```python
from build123d import *

# Parameters (mm, degrees)
F0_W     = 431.8
F0_H     = 228.6
F1_DEPTH = 12.7
F3_DEPTH = 22.225
F4_W     = 3.175
F4_H     = 12.7
F5_DEPTH = 203.2


with BuildPart() as f1:
    # F0 (on Front) → F1 (new body)
    with BuildSketch(Plane.XZ):
        with Locations((215.9, 114.3)):
            Rectangle(F0_W, F0_H)
    extrude(amount=F1_DEPTH)

    # F2 (on face) → F3 (join)
    with BuildSketch(Plane.XZ.offset(12.7)):
        Polygon((139.7, 107.95), (139.7, 114.3), (139.7, 120.65), (114.3, 120.65), (114.3, 114.3), (114.3, 107.95), align=None)
        Polygon((317.5, 120.65), (292.1, 120.65), (292.1, 114.3), (292.1, 107.95), (317.5, 107.95), (317.5, 114.3), align=None)
    extrude(amount=F3_DEPTH)

    # F4 (on face) → F5 (join, through all)
    with BuildSketch(Plane.YZ.offset(317.5)):
        with Locations((-36.5125, 114.3)):
            Rectangle(F4_W, F4_H)
    extrude(amount=-F5_DEPTH)


solid = f1.part
```
The listing builds one solid part. Answer for the finished solid, in the listing's coordinates (mm). A direction names the side the tool comes from. Give positions to 0.01 mm unless a question says otherwise; leave off trailing zeros. Order: outer loops, then holes, each group sorted by start corner. A loop starts at its lowest first (then second) coordinate and runs counter-clockwise, first axis right, second up.
Item 1: For a pull along X with two mould halves and no side action, classify faces 1 (the face through (317.5, -26, 114)), 2 (the face through (139.7, -24, 114)), 3 (the face through (213, 0, 116)) as pulls with the +X half, pulls with the -X half, needs draft (parallel to the pull), parting line crosses it, or undercut.
From the geometry:
face 1: pulls with the +X half
face 2: undercut
face 3: needs draft
Item 2: The part is cut by section A-A, the plane x = 283.5. Give the vertices of the cut face in (y, z) (3 decimals).
From the geometry:
outline: (-38.1, 107.95) - (-34.925, 107.95) - (-34.925, 120.65) - (-38.1, 120.65) - close; (-12.7, 0) - (0, 0) - (0, 228.6) - (-12.7, 228.6) - close
Item 3: The part is cut by section D-D, the plane x = 36.5. Give the vertices of the cut face in (y, z).
From the geometry:
outline: (-12.7, 0) - (0, 0) - (0, 228.6) - (-12.7, 228.6) - close
Item 4: Find the intervals of material crossed by probe 1 along Y at (x, z) = (371, 37); probe 2 along X at (y, z) = (-35, 115.5), in increasing order.
From the geometry:
probe 1: y = -12.7 to 0
probe 2: x = 114.3 to 317.5
Item 5: Given pin 1 Ø6 at (x, z) = (62.5, 174) entering from -Y; pin 2 Ø10 at (y, z) = (-27, 113) entering from -X; pin 3 Ø4 at (y, z) = (-27.5, 113) entering from +X; pin 4 Ø12.5 at (x, y) = (177, -25.5) entering from -Z, each flat-ended and moving along its own axis, determine where each tip first touches the part or whether it passes through.
From the geometry:
pin 1: stops at y = -12.7
pin 2: stops at x = 114.3
pin 3: stops at x = 317.5
pin 4: passes through
Item 6: The part is cut by section B-B, the plane y = -27. Give the vertices of the cut face in (x, z).
From the geometry:
outline: (114.3, 107.95) - (139.7, 107.95) - (139.7, 120.65) - (114.3, 120.65) - close; (292.1, 107.95) - (317.5, 107.95) - (317.5, 120.65) - (292.1, 120.65) - close
Item 7: The part is cut by section C-C, the plane z = 45.5. Give the vertices of the cut face in (x, y).
From the geometry:
outline: (0, -12.7) - (431.8, -12.7) - (431.8, 0) - (0, 0) - close
Item 8: Which of the six approach directions +Z, -Z, +X, -X, +Y, -Y give full straight-line access (tool end or side, diameter ignored) to faces 4 (the face through (114.3, -26, 114)), 5 (the face through (292.1, -24, 114)), 6 (the face through (216, -36, 120.65)), 7 (the face through (216, -36, 107.95))?
From the geometry:
face 4: +Z, -Z, -X, -Y
face 5: +Z, -Z
face 6: +Z, +X, -X, -Y
face 7: -Z, +X, -X, -Y
